Autodesk Inventor part; units mm, degrees
ref_plane "YZ Plane" through (0, 0, 0) normal (1, 0, 0) x (0, 1, 0)
ref_plane "XZ Plane" through (0, 0, 0) normal (0, 1, 0) x (-1, 0, 0)
ref_plane "XY Plane" through (0, 0, 0) normal (0, 0, 1) x (1, 0, 0)
sketch "Sketch1" plane through (0, 0, 0) normal (0, 1, 0) x (-1, 0, 0)
  circle A0 centre (0, 0) radius 135
  circle A1 centre (0, 0) radius 110
  dimension "d0" = 270
  dimension "d1" = 220
extrude "Extrusion1" add sketch "Sketch1" along normal blind 55
sketch "Sketch2" plane through (0, 0, 0) normal (0, 0, 1) x (1, 0, 0)
  circle A0 centre (0, 5) radius 18
  line L0 (135, 0) -> (-135, 0)
  point P0 (0, 0)
  dimension "d4" = 36
  dimension "d5" = 5
extrude "Extrusion2" cut sketch "Sketch2" against normal through all
sketch "Sketch3" plane through (0, 0, 0) normal (0, -1, 0) x (1, 0, 0)
  circle A0 centre (0, 0) radius 140
extrude "Extrusion3" cut sketch "Sketch3" against normal blind 20
sketch "Sketch4" plane through (0, 20, 0) normal (0, -1, 0) x (1, 0, 0)
  line L0 (0, 0) -> (70, 0)
  line L1 (80, -100) -> (60, -100)
  line L2 (60, -100) -> (60, 100)
  line L3 (60, 100) -> (80, 100)
  line L4 (80, 100) -> (80, -100)
  line L5 (80, -100) -> (60, 100) construction
  line L6 (60, -100) -> (80, 100) construction
  dimension "d10" = 70
  dimension "d11" = 20
  dimension "d12" = 200
extrude "Extrusion4" cut sketch "Sketch4" against normal through all
sketch "Sketch5" plane through (0, 55, 0) normal (0, 1, 0) x (1, 0, 0)
  circle A0 centre (0, 0) radius 127.5
  circle A1 centre (127.5, 0) radius 2
  circle A2 centre (103.1497, 74.9426) radius 2
  circle A3 centre (39.3997, 121.2597) radius 2
  circle A4 centre (-39.3997, 121.2597) radius 2
  circle A5 centre (-103.1497, 74.9426) radius 2
  circle A6 centre (-127.5, 0) radius 2
  circle A7 centre (-103.1497, -74.9426) radius 2
  circle A8 centre (-39.3997, -121.2597) radius 2
  circle A9 centre (39.3997, -121.2597) radius 2
  circle A10 centre (103.1497, -74.9426) radius 2
  dimension "d15" = 255
  dimension "d16" = 4
  dimension "d19" = 360
hole "Hole1" at (127.5, 55, 0) at (103.1497, 55, 74.9426) at (39.3997, 55, 121.2597) at (-39.3997, 55, 121.2597) at (-103.1497, 55, 74.9426) at (-127.5, 55, 0) at (-103.1497, 55, -74.9426) at (-39.3997, 55, -121.2597) at (39.3997, 55, -121.2597) at (103.1497, 55, -74.9426) direction (0, -1, 0) diameter 5 end through all
sketch "Sketch6" plane through (0, 55, 0) normal (0, 1, 0) x (1, 0, 0)
  circle A0 centre (0, 0) radius 140
extrude "Extrusion5" cut sketch "Sketch6" against normal blind 15
sketch "Sketch7" plane through (0, 40, 0) normal (0, 1, 0) x (1, 0, 0)
  circle A0 centre (0, 0) radius 140
  line L0 (80, -100) -> (80, -75.4983)
  line L1 (80, -100) -> (80, -75.4983)
  line L2 (60, -100) -> (80, -100)
  line L3 (80, -100) -> (60, -100)
  line L4 (60, -100) -> (60, -92.1954)
  line L5 (60, 100) -> (60, 92.1954)
  line L6 (60, 92.1954) -> (60, 100)
  line L7 (60, 100) -> (80, 100)
  line L8 (80, 100) -> (80, 75.4983)
  arc A1 (80, -75.4983) -> (80, 75.4983) centre (0, 0) ccw
  arc A2 (60, 92.1954) -> (60, -92.1954) centre (0, 0) ccw
  arc A3 (-25, -65) -> (25, -65) centre (0, -65) ccw
  arc A4 (25, 65) -> (-25, 65) centre (0, 65) ccw
  arc A5 (25, -27.9508) -> (25, 27.9508) centre (0, 0) ccw
  arc A6 (-25, 27.9508) -> (-25, -27.9508) centre (0, 0) ccw
  line L9 (25, 65) -> (25, 27.9508)
  line L10 (25, -27.9508) -> (25, -65)
  line L11 (-25, -65) -> (-25, -27.9508)
  line L12 (-25, 27.9508) -> (-25, 65)
extrude "Extrusion6" add sketch "Sketch7" against normal blind 1 contours L2 L4 A2 L5 L7 L8 A1 L0
sketch "Sketch8" plane through (0, 39, 0) normal (0, -1, 0) x (1, 0, 0)
  line L0 (80, -75.4983) -> (80, -100)
  line L1 (80, -100) -> (60, -100)
  line L2 (60, -100) -> (60, 100)
  line L3 (60, 100) -> (80, 100)
  line L4 (80, 100) -> (80, 75.4983)
  line L5 (80, -75.4983) -> (80, -100)
  arc A0 (80, -75.4983) -> (80, 75.4983) centre (0, 0) ccw
  arc A1 (60, 92.1954) -> (60, -92.1954) centre (0, 0) ccw
extrude "Extrusion7" add sketch "Sketch8" along normal blind 14 contours L0 L1 L2 L3 L4 A0
sketch "Sketch9" plane through (0, 20, 0) normal (0, -1, 0) x (1, 0, 0)
  arc A0 (9.9499, -134.6328) -> (-9.9499, -134.6328) centre (0, 0) ccw
  spline S0 degree 7 poles (9.9499, -134.6328) (9.4556, -134.6694) (8.9421, -134.7052) (8.4096, -134.74) (7.8582, -134.7735) (7.2882, -134.8052) (6.6998, -134.835) (5.2633, -134.8999) (4.3998, -134.933) (3.5087, -134.9604) (2.5962, -134.9814) (1.6691, -134.9951) (0.7345, -135.0012) (-1.7136, -134.9976) (-3.2083, -134.9756) (-4.6621, -134.9347) (-6.0536, -134.8776) (-7.364, -134.8084) (-8.5782, -134.7318) (-9.7236, -134.6494) (-9.7616, -134.6466) (-9.7995, -134.6439) (-9.8372, -134.6411) (-9.8749, -134.6384) (-9.9124, -134.6356) (-9.9499, -134.6328) knots 0 0 0 0 0 0 0 0 0.214533 0.214533 0.214533 0.214533 0.214533 0.214533 0.508291 0.508291 0.508291 0.508291 0.508291 0.508291 0.983641 0.983641 0.983641 0.983641 0.983641 0.983641 1 1 1 1 1 1 1 1
  line L0 (0, 135) -> (0, -135)
  line L1 (132.949, -23.4425) -> (-132.949, 23.4425)
  point P0 (0, 0)
  dimension "d40" = 80
extrude "Extrusion8" cut sketch "Sketch9" against normal through all contours S0 L0 L1 A0 | S0 A0 L1 L0 | L0 L1 A0 picked at (-5.2242, 89.6957)
sketch "Sketch10" plane through (0, 20, 110) normal (-1, 0, 0) x (0, 0, 1)
  line L0 (25, 0) -> (-133.4425, 0)
  line L1 (22.5, 0) -> (40, 0)
  line L2 (45, 5) -> (45, 15)
  line L3 (40, 20) -> (22.5, 20)
  line L4 (22.5, 20) -> (22.5, 0)
  line L5 (25, 20) -> (25, 0)
  arc A0 (40, 0) -> (45, 5) centre (40, 5) ccw
  arc A1 (45, 15) -> (40, 20) centre (40, 15) ccw
  point P0 (-110, -20)
  point P1 (45, 20)
  point P2 (45, 0)
  dimension "d43" = 22.5
  dimension "d44" = 20
  dimension "d45" = 20
  dimension "d46" = 5
extrude "Extrusion9" add sketch "Sketch10" against normal blind 10
sketch "Sketch11" plane through (132.949, 20, -23.4425) normal (-0.1736482, 0, -0.9848078) x (-0.9848078, 0, 0.1736482)
  line L0 (0, 20) -> (97.5, 20)
  line L1 (2.5, 20) -> (-15, 20)
  line L2 (-20, 15) -> (-20, 5)
  line L3 (-15, 0) -> (2.5, 0)
  line L4 (2.5, 0) -> (2.5, 20)
  line L5 (0, 0) -> (0, 20)
  arc A0 (-20, 5) -> (-15, 0) centre (-15, 5) ccw
  arc A1 (-15, 20) -> (-20, 15) centre (-15, 15) ccw
  point P0 (135, -20)
  point P1 (-20, 0)
  point P2 (-20, 20)
  dimension "d49" = 22.5
  dimension "d50" = 20
  dimension "d51" = 20
  dimension "d52" = 5
extrude "Extrusion10" add sketch "Sketch11" against normal blind 10
fillet "Fillet1" radius 2.5 2 edges at (10, 30, 134.6291) (134.3203, 30, -13.53)
sketch "Sketch12" plane through (10, 20, 110) normal (1, 0, 0) x (0, 0, -1)
  line L0 (-40, 0) -> (-26.9306, 0)
  line L1 (-45, 15) -> (-45, 5)
  point P0 (110, -20)
  point P1 (-35, 10)
  dimension "d56" = 10
  dimension "d57" = 10
hole "Hole2" at (10, 30, 145) direction (-1, 0, 0) diameter 8.2 end through all counterbore diameter 13.2 counterbore depth 6
sketch "Sketch13" plane through (134.6855, 20, -13.5944) normal (0.1736482, 0, 0.9848078) x (0.9848078, 0, -0.1736482)
  line L0 (16.6, 7.2662) -> (12.7338, 3.4)
  line L1 (12.7338, 3.4) -> (7.2662, 3.4)
  line L2 (7.2662, 3.4) -> (3.4, 7.2662)
  line L3 (3.4, 7.2662) -> (3.4, 12.7338)
  line L4 (3.4, 12.7338) -> (7.2662, 16.6)
  line L5 (7.2662, 16.6) -> (12.7338, 16.6)
  line L6 (12.7338, 16.6) -> (16.6, 12.7338)
  line L7 (16.6, 12.7338) -> (16.6, 7.2662)
  line L8 (20, 5) -> (20, 15)
  line L9 (1.9306, 0) -> (15, 0)
  point P0 (-135, -20)
  point P1 (10, 10)
  point P2 (20, 10)
  dimension "d65" = 10
  dimension "d66" = 10
  dimension "d67" = 13.2
extrude "Extrusion11" cut sketch "Sketch13" against normal blind 6
sketch "Sketch14" plane through (133.6436, 20, -19.5033) normal (0.1736482, 0, 0.9848078) x (0.9848078, 0, -0.1736482)
  line L0 (1.9306, 0) -> (15, 0)
  line L1 (20, 5) -> (20, 15)
  point P0 (-135, -20)
  point P1 (10, 10)
  dimension "d70" = 10
  dimension "d71" = 10
hole "Hole3" at (143.4917, 30, -21.2398) direction (-0.1736482, 0, -0.9848078) diameter 8.2 end through all
properties part number "Cylinder Spacer Top_Q3"
Can you work these out from the model? Positions are in its coordinate system, mm. A direction names the side the tool comes from. Coordinates: 2 decimals unless noted, no trailing zeros. Loops run counter-clockwise (first coordinate to the right, second up) from the corner with the lowest first, then second, coordinate; pieces in that order, holes last.
1) I need wall thicknesses on probe 1 along Y at (x, z) = (1.95, 145); probe 2 along Y at (x, z) = (107.5, 7.5); probe 3 along Z at (x, y) = (39, 31). Which ranges of each line are inside material? Lowest first, please.
2) Imagine slicing it at D-D on z = 45. List the corners of the cut face in (x, y) for me, plus the area to 3 significant figures.
3) Imagine slicing it at B-B on y = 30. State how many separate pieces and enclosed holes the cut face has, plus the area to 3 significant figures.
4) Imagine slicing it at A-A on z = 145. List the corners of the cut face in (x, y) for me.
5) Imagine slicing it at C-C on x = 127.5. List the corners of the cut face in (y, z) for me.
6) For pin 1 (1.5 mm diameter, centred on x = 65, y = 22.5, fed in from -Z); pin 2 (5.5 mm diameter, centred on y = 27, z = 142.5, fed in from +X); pin 3 (4 mm diameter, centred on y = 30, z = 144.5, fed in from +X); pin 4 (15 mm diameter, centred on x = 86, z = 30, fed in from -Y), each with a flat end and sliding along its axis, tell me the tip position at first contact or that it passes through.
7) Which directions (+Z, -Z, +X, -X, +Y, -Y) give clear straight access to the entire face, cutting with the end or side of a thin tool? Please do faces 1 (the flat face through (140.512, 33.026, -20.716)), 2 (the flat face through (36, 39, 62)), 3 (the cylindrical face through (1.972, 29.82, 149.096)), 4 (the flat face through (148.589, 34.694, -19.051)), 5 (the flat face through (4, 34.3, 145.1)).
8) Thinking about a two-plate mould opening in X: for faces 6 (the flat face through (70, 22, 100)), 7 (the cylindrical face through (31.719, 29.367, 105.328)), 8 (the flat face through (139.4, 34.64, -17.43)), 9 (the cylindrical face through (152.021, 38.574, -21.799)), which applies, pulls with the +X half, pulls with the -X half, needs draft (parallel to the pull), parting line crosses it, or undercut?
Completed:
1. probe 1: y = 20 to 25.9, 34.1 to 40
1. probe 2: y = 25 to 40
1. probe 3: z = 102.85 to 118.79, 123.73 to 129.24
2. outline: (25, 39) - (60, 39) - (60, 25) - (100.37, 25) - (100.37, 20) - (127.28, 20) - (127.28, 40) - (25, 40) - close
2. area: 1,180 mm2
3. separate pieces: 3
3. enclosed holes: 3
3. area: 9,450 mm2
4. outline: (0, 20) - (10, 20) - (10, 23.4) - (4, 23.4) - (4, 25.9) - (0, 25.9) - close; (0, 34.1) - (4, 34.1) - (4, 36.6) - (10, 36.6) - (10, 40) - (0, 40) - close
5. outline: (20, -22.48) - (40, -22.48) - (40, -2.5) - (20, -2.5) - close; (20, 2.5) - (40, 2.5) - (40, 44.37) - (20, 44.37) - close
6. pin 1: stops at z = 100
6. pin 2: stops at x = 10
6. pin 3: passes through
6. pin 4: stops at y = 25
7. face 1: none
7. face 2: -Z, -X, -Y
7. face 3: +X, -X
7. face 4: +Z
7. face 5: +X
8. face 6: undercut
8. face 7: pulls with the -X half
8. face 8: undercut
8. face 9: pulls with the +X half
